Check sheet for the drawn part. Datum: minimum x, y, z corner. Units: mm. A direction names the side the tool comes from. Coordinates: 2 decimals unless noted, no trailing zeros. Order: outer loops, then holes, each group sorted by start corner. A loop starts at its lowest first (then second) coordinate and runs counter-clockwise, first axis right, second up. Notation, with made-up numbers: (69, -40) - (112, -40) arc R23 cw to (112, -4) - close; hole circle Ø9 at (-2, 67). An arc over 180 degrees is marked (long way). Answer as CSV lines item,"result". Start each with the question number.
1. Section check D-D (z = 0.5). Record the cut outline in (x, y), and give its area (3 significant figures).
2. Go/stop test with a flat-tipped pin: pin 1 (5 mm diameter, centred on x = 18.5, z = 3, fed in from +Y). Record where the tip stops, or that it passes through.
3. Section check B-B (y = 25). Record the cut outline in (x, z), and give its area (3 significant figures).
4. Section check C-C (y = 18). Record the cut outline in (x, z), and give its area (3 significant figures).
5. Section check A-A (z = 5). Record the cut outline in (x, y).
6. Mould release check, pull along Z, two halves, no side actions. Record for the marked faces 1, 2 and 3: pulls with the +Z half, pulls with the -Z half, needs draft (parallel to the pull), parting line crosses it, or undercut.
7. Set-up check for the marked faces 4, 5 and 6: record each of +Z, -Z, +X, -X, +Y, -Y from which the full face is reachable in a straight line by a thin tool's end or side.
8. Material ranges on L1, parallel to X at y = 12, z = 2.25; L2, parallel to Y at x = 33.9, z = 5; L3, parallel to Y at x = 2.3, z = 5, recorded low to high. Write a range as [from, to].
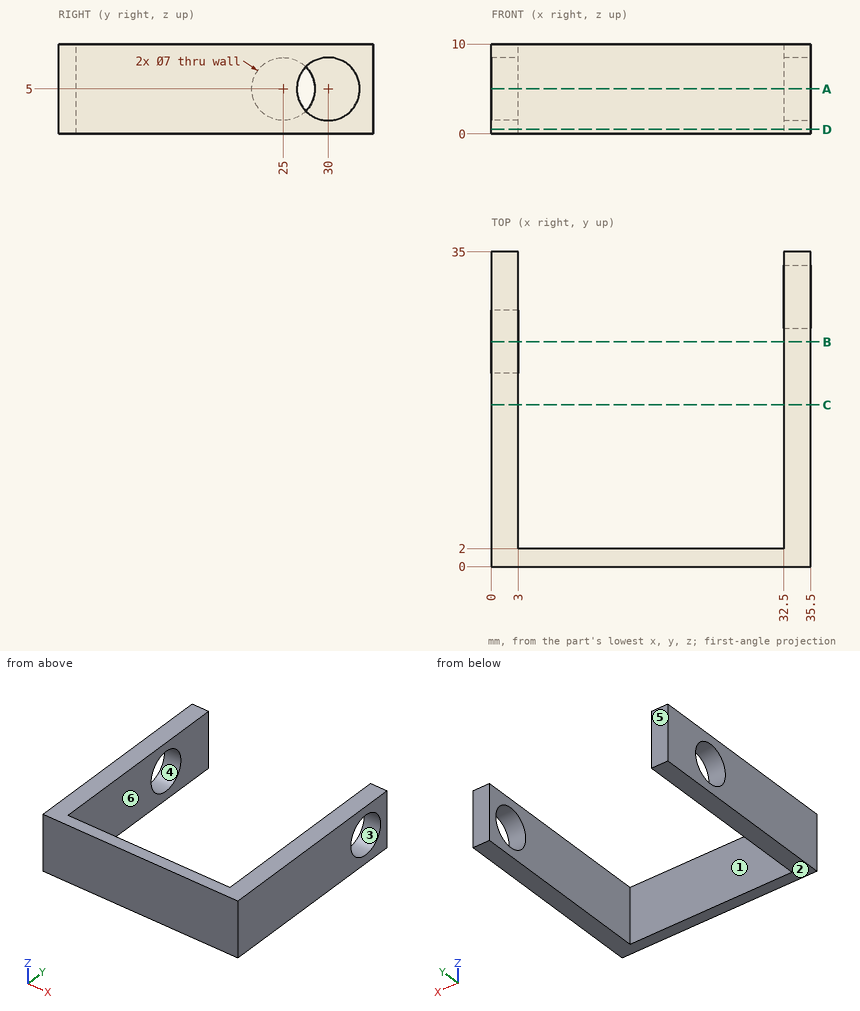
Evaluation:
1,outline,"(0, 0) - (35.5, 0) - (35.5, 35) - (32.5, 35) - (32.5, 2) - (3, 2) - (3, 35) - (0, 35) - close"
1,area,"269 mm²"
2,pin 1,"stops at y = 2"
3,outline,"(0, 0) - (3, 0) - (3, 1.5) - (0, 1.5) - close; (0, 8.5) - (3, 8.5) - (3, 10) - (0, 10) - close; (32.5, 0) - (35.5, 0) - (35.5, 10) - (32.5, 10) - close"
3,area,"39.0 mm²"
4,outline,"(0, 0) - (3, 0) - (3, 10) - (0, 10) - close; (32.5, 0) - (35.5, 0) - (35.5, 10) - (32.5, 10) - close"
4,area,"60.0 mm²"
5,outline,"(0, 0) - (35.5, 0) - (35.5, 26.5) - (32.5, 26.5) - (32.5, 2) - (3, 2) - (3, 21.5) - (0, 21.5) - close; (0, 28.5) - (3, 28.5) - (3, 35) - (0, 35) - close; (32.5, 33.5) - (35.5, 33.5) - (35.5, 35) - (32.5, 35) - close"
6,face 1,"needs draft"
6,face 2,"pulls with the -Z half"
6,face 3,"undercut"
7,face 4,"-X"
7,face 5,"+Z, -Z, +X, -X, +Y"
7,face 6,"+Z, -Z, +Y"
8,L1,"x = [0, 3], [32.5, 35.5]"
8,L2,"y = [0, 26.5], [33.5, 35]"
8,L3,"y = [0, 21.5], [28.5, 35]"
